Part model, mm, in its own coordinate system. Face numbers are marked on the shaded views. A direction names the side the tool comes from. Round coordinates to 2 decimals unless told otherwise and drop trailing zeros. Loops run counter-clockwise (first coordinate to the right, second up) from the corner with the lowest first, then second, coordinate; pieces in that order, holes last. Notation, with made-up numbers: M 14,73.25 L 42,73.25 A19 ccw 42,84.25 Z; hole C 35,-24 d2. An arc over 180 degrees is marked long. Answer as CSV lines item,"result". Start each with the question number.
Item 1: Band-saw the part on D-D (z = 0.5). Give the cut face in (x, y), and give its area (3 significant figures).
Item 2: Band-saw the part on C-C (z = -14.25). Give the cut face in (x, y).
Item 3: Which spindle directions (+Z, -Z, +X, -X, +Y, -Y) get a long thin tool onto all of the face, cutting with end or side? Do the marked faces 1 and 2. Say none if no direction does.
Item 4: Wall check: line 1 (Z direction, x = -3.25, y = -2.25); line 2 (Z direction, x = -3.25, y = -0.75); line 3 (X direction, y = -2, z = -6.5). Give the ranges that are in metal, low to high.
Item 5: Drop flat-ended pins along their axis: pin 1 Ø2 at (x, z) = (2, -7) entering from +Y; pin 2 Ø5 at (y, z) = (-3, -10.5) entering from +X; pin 3 Ø2 at (y, z) = (0, -3.5) entering from +X. Give the stop position or say it passes through.
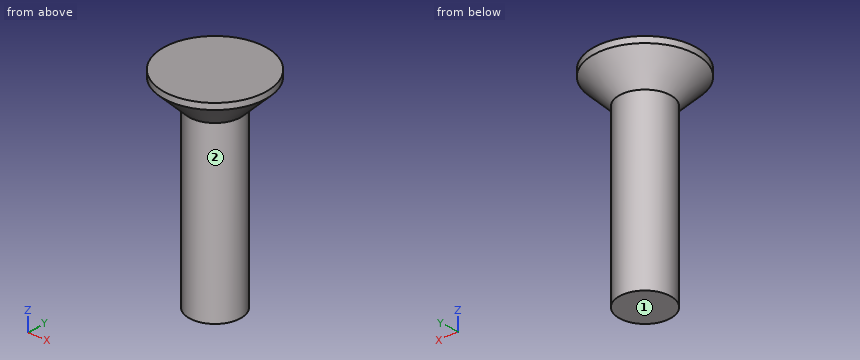
Autodesk Inventor part; units mm, degrees
ref_plane "YZ Plane" through (0, 0, 0) normal (1, 0, 0) x (0, 1, 0)
ref_plane "XZ Plane" through (0, 0, 0) normal (0, 1, 0) x (-1, 0, 0)
ref_plane "XY Plane" through (0, 0, 0) normal (0, 0, 1) x (1, 0, 0)
sketch "スケッチ1" plane through (0, 0, 0) normal (0, 0, 1) x (1, 0, 0)
  circle A0 centre (0, 0) radius 5
  dimension "d0" = 10
extrude "押し出し1" add sketch "スケッチ1" along normal blind 3.1
sketch "スケッチ2" plane through (0, 0, 3.1) normal (0, 0, 1) x (1, 0, 0)
  circle A0 centre (0, 0) radius 2.5
  dimension "d3" = 5
extrude "押し出し2" add sketch "スケッチ2" against normal blind 20
chamfer "面取り1" distance 2.5 angle 45 1 edges at (-5, 0, 0)
thread "ねじ1"
properties part number "ネジ皿m5,20" material "鋼、高強度、低合金"
Answer block:
1,outline,"C 0,0 d6"
1,area,"28.3 mm^2"
2,outline,"C 0,0 d5"
3,face 1,"-Z, +X, -X, +Y, -Y"
3,face 2,"-Z"
4,line 1,"z = 1.45 to 3.1"
4,line 2,"z = 0.83 to 3.1"
4,line 3,"x = -1.5 to 1.5"
5,pin 1,"stops at y = 2.29"
5,pin 2,"stops at x = 2.45"
5,pin 3,"stops at x = 2.5"
